The listing builds one solid part. Answer for the finished solid, in the listing's coordinates (mm). A direction names the side the tool comes from. Coordinates: 2 decimals unless noted, no trailing zeros. Order: outer loops, then holes, each group sorted by start corner. A loop starts at its lowest first (then second) coordinate and runs counter-clockwise, first axis right, second up. Notation, with made-up numbers: (-13.75, 54.25) -> (0.25, 54.25) arc R36 ccw to (0.25, 89.25) -> close; hole circle Ø5 at (32.25, -31.5). An arc over 180 degrees is marked (long way). Return JSON: item names as keys, results as strings.
```python
from build123d import *

# Parameters (mm, degrees)
SKETCH1_W           = 50
SKETCH1_H           = 1.5
BOSS_EXTRUDE1_DEPTH = 50
CUT_EXTRUDE1_DEPTH  = 1.5
BOSS_EXTRUDE2_DEPTH = 1.5


with BuildPart() as part:
    # Sketch1 → Boss-Extrude1 (new body)
    with BuildSketch(Plane.XY):
        with Locations((0, -1.811768481)):
            Rectangle(SKETCH1_W, SKETCH1_H)
    extrude(amount=BOSS_EXTRUDE1_DEPTH)

    # Sketch2 → Cut-Extrude1 (cut)
    with BuildSketch(Plane(origin=(0, -1.061768481, 0), x_dir=(1, 0, 0), z_dir=(0, 1, 0))):
        with BuildLine():
            Line((-10, -36.633249581), (-10, -50))
            Line((-10, -50), (10, -50))
            Line((10, -50), (10, -36.633249581))
            ThreePointArc((10, -36.633249581), (0, -18), (-10, -36.633249581))
        make_face()
    extrude(amount=-CUT_EXTRUDE1_DEPTH, mode=Mode.SUBTRACT)

    # Sketch4 → Boss-Extrude2 (add)
    with BuildSketch(Plane.ZY.offset(25)):
        Polygon((0, -2.561768481), (0, -17.561768481), (30, -2.561768481), align=None)
    boss_extrude2 = extrude(amount=-BOSS_EXTRUDE2_DEPTH)

    # Mirror1: Boss-Extrude2 across plane
    add(boss_extrude2.mirror(Plane(origin=(0, 0, 0), x_dir=(0, 0, 1), z_dir=(1, 0, 0))))


solid = part.part
```
Item 1: The part is cut by section D-D on z = 9. Determine the outline of the cut face in (x, y), plus the area to 4 significant figures.
Answer list:
{"outline": "(-25, -13.06) -> (-23.5, -13.06) -> (-23.5, -2.56) -> (23.5, -2.56) -> (23.5, -13.06) -> (25, -13.06) -> (25, -1.06) -> (-25, -1.06) -> close", "area": "106.5 mm2"}
Item 2: The part is cut by section B-B on y = -16. Determine the outline of the cut face in (x, z), plus the area to 3 significant figures.
Answer list:
{"outline": "(-25, 0) -> (-23.5, 0) -> (-23.5, 3.12) -> (-25, 3.12) -> close; (23.5, 0) -> (25, 0) -> (25, 3.12) -> (23.5, 3.12) -> close", "area": "9.37 mm2"}
Item 3: Which of the six approach directions +Z, -Z, +X, -X, +Y, -Y give full straight-line access (tool end or side, diameter ignored) to faces 5 (the flat face through (-25, -6, 14)), 6 (the flat face through (10, -2, 43)), 7 (the flat face through (23.5, -8, 11))?
Answer list:
{"face 5": "+Z, -Z, -X, +Y, -Y", "face 6": "+Z, +Y, -Y", "face 7": "+Z, -Z, -Y"}
Item 4: The part is cut by section C-C on x = 18.5. Determine the outline of the cut face in (y, z), plus the area to 3 significant figures.
Answer list:
{"outline": "(-2.56, 0) -> (-1.06, 0) -> (-1.06, 50) -> (-2.56, 50) -> close", "area": "75.0 mm2"}
Item 5: The part is cut by section A-A on z = 38. Determine the outline of the cut face in (x, y), plus the area to 3 significant figures.
Answer list:
{"outline": "(-25, -2.56) -> (-10, -2.56) -> (-10, -1.06) -> (-25, -1.06) -> close; (10, -2.56) -> (25, -2.56) -> (25, -1.06) -> (10, -1.06) -> close", "area": "45.0 mm2"}
Item 6: Find the intervals of material crossed by probe 1 along X at (y, z) = (-2.1, 30); probe 2 along Y at (x, z) = (3, 17); probe 3 along X at (y, z) = (-10.5, 3), in increasing order.
Answer list:
{"probe 1": "-25 to -12, 12 to 25", "probe 2": "-2.56 to -1.06", "probe 3": "-25 to -23.5, 23.5 to 25"}
Item 7: A flat-ended cylindrical pin translates along its axis: pin 1 (4 mm diameter, centred on x = 16.5, z = 20.5, fed in from -Y). Find the tip coordinate at first contact, or state that the pin passes through.
Answer list:
{"pin 1": "y = -2.56"}
Item 8: Determine the mould class of faces 1 (the cylindrical face through (0, -2, 18)), 2 (the flat face through (17, -2, 50)), 3 (the flat face through (0, -2, 0)), 4 (the flat face through (-6, -1.062, 19)) for opening direction Z: pulls with the +Z half, pulls with the -Z half, needs draft (parallel to the pull), parting line crosses it, or undercut.
Answer list:
{"face 1": "undercut", "face 2": "pulls with the +Z half", "face 3": "pulls with the -Z half", "face 4": "needs draft"}
